Check sheet for the modelled part. Datum: model origin and axes. Units: mm. Face numbers are marked on the shaded views. A direction names the side the tool comes from. Give positions to 0.01 mm unless a question says otherwise; leave off trailing zeros. Write each loop counter-clockwise with the first axis right and the second up, starting at its lowest first coordinate (ties: lowest second). Pieces come first, ordered by that corner, then holes.
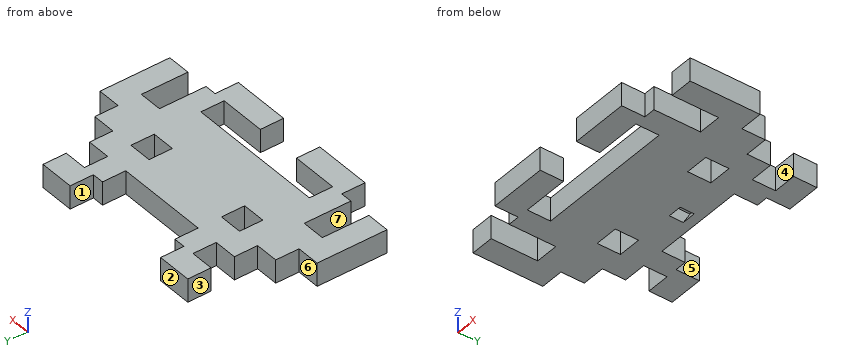
from build123d import *

# Parameters (mm, degrees)
F0_W     = 10
F0_H     = 10
F0_R     = 6
F1_DEPTH = 10
F3_DEPTH = 3


with BuildPart() as f1:
    # F0 (on Top) → F1 (new body)
    with BuildSketch(Plane.XY):
        Polygon((10, 0), (0, 0), (-10, 0), (-20, 0), (-20, 10), (-25, 10), (-30, 10), (-30, 0), (-40, 0), (-40, -10), (-50, -10), (-50, -20), (-60, -20), (-60, -30), (-60, -50), (-50, -50), (-50, -30), (-40, -30), (-40, -40), (-40, -50), (-35, -50), (-30, -50), (-30, -40), (-20, -40), (-10, -40), (0, -40), (10, -40), (20, -40), (30, -40), (30, -50), (35, -50), (40, -50), (40, -40), (40, -30), (50, -30), (50, -50), (60, -50), (60, -30), (60, -20), (50, -20), (50, -10), (40, -10), (40, 0), (30, 0), (30, 10), (25, 10), (20, 10), (20, 0), align=None)
        with Locations((-25, -15)):
            Rectangle(F0_W, F0_H, mode=Mode.SUBTRACT)
        with Locations((0, -12)):
            Circle(F0_R, mode=Mode.SUBTRACT)
        with Locations((25, -15)):
            Rectangle(F0_W, F0_H, mode=Mode.SUBTRACT)
        Polygon((-30, 10), (-25, 10), (-25, 20), (-30, 20), (-40, 20), (-40, 10), align=None)
        Polygon((25, 20), (25, 10), (30, 10), (40, 10), (40, 20), (30, 20), align=None)
        Polygon((-30, -50), (-35, -50), (-35, -60), (-10, -60), (-10, -50), align=None)
        Polygon((35, -60), (35, -50), (30, -50), (10, -50), (10, -60), align=None)
        with Locations((0, -12)):
            Circle(F0_R)
    extrude(amount=F1_DEPTH)

    # F2 (on Right) → F3 (cut, symmetric)
    with BuildSketch(Plane.YZ):
        Polygon((-10, 5), (-10, 0), (-4, 0), (-1.1132486541, 5), align=None)
    extrude(amount=F3_DEPTH, both=True, mode=Mode.SUBTRACT)


solid = f1.part
1) Sectioned sample at C-C on y = -44. Record the boundary of the cut face in (x, z), then the cut area to 3 significant figures.
2) Access from +Z, -Z, +X, -X, +Y, -Y to the whole of each face (thin tool, end or side, straight path). Record for the marked faces 4, 5, 6 and 7.
3) Sectioned sample at A-A on y = 11.5. Record the boundary of the cut face in (x, z), then the cut area to 3 significant figures.
4) Sectioned sample at B-B on x = 38. Record the boundary of the cut face in (y, z), then the cut area to 3 significant figures.
5) Draft check along X on the marked faces 1, 2 and 3. Enter one of: +X half, -X half, draft (parallel to the pull), parting line (faces both ways), or undercut.
6) Gauge pin test, flat ends, axial feed: pin 1 (3 mm diameter, centred on y = -16.5, z = 5.5, fed in from +X); pin 2 (4 mm diameter, centred on y = -6.5, z = 3, fed in from +X); pin 3 (2.5 mm diameter, centred on x = 22, z = 7.5, fed in from +Y); pin 4 (6 mm diameter, centred on x = 5.5, y = -22, fed in from -Z). Record the tip position at first contact, or that the pin passes through.
7) Scan lines: L1, parallel to X at y = -14.5, z = 8.25; L2, parallel to X at y = -38, z = 1; L3, parallel to X at y = -49.5, z = 0.5. Record each from-to range of solid material in increasing order.
8) Sectioned sample at D-D on y = -35. Record the boundary of the cut face in (x, z), then the cut area to 3 significant figures.
Answers below:
1. outline: (-60, 0) - (-50, 0) - (-50, 10) - (-60, 10) - close; (-40, 0) - (-30, 0) - (-30, 10) - (-40, 10) - close; (30, 0) - (40, 0) - (40, 10) - (30, 10) - close; (50, 0) - (60, 0) - (60, 10) - (50, 10) - close
1. area: 400 mm2
2. face 4: +Z, -Z, +X
2. face 5: +Z, -Z, +Y
2. face 6: +Z, -Z, -X, +Y
2. face 7: +Z, -Z, -Y
3. outline: (-40, 0) - (-25, 0) - (-25, 10) - (-40, 10) - close; (25, 0) - (40, 0) - (40, 10) - (25, 10) - close
3. area: 300 mm2
4. outline: (-50, 0) - (0, 0) - (0, 10) - (-50, 10) - close; (10, 0) - (20, 0) - (20, 10) - (10, 10) - close
4. area: 600 mm2
5. face 1: undercut
5. face 2: draft
5. face 3: -X half
6. pin 1: stops at x = 50
6. pin 2: stops at x = 40
6. pin 3: stops at y = 10
6. pin 4: stops at z = 0
7. L1: x = -50 to -30, -20 to 20, 30 to 50
7. L2: x = -60 to -50, -40 to 40, 50 to 60
7. L3: x = -60 to -50, -40 to -30, 30 to 40, 50 to 60
8. outline: (-60, 0) - (-50, 0) - (-50, 10) - (-60, 10) - close; (-40, 0) - (40, 0) - (40, 10) - (-40, 10) - close; (50, 0) - (60, 0) - (60, 10) - (50, 10) - close
8. area: 1,000 mm2
